```python
from build123d import *

# Parameters (mm, degrees)
F0_R     = 43.5
F0_R_2   = 41
F1_DEPTH = 14
F0_R_3   = 46.5412209473
F2_DEPTH = 2.5
F3_R     = 1.24999


# Not quite as in the source:
# - a fillet or chamfer is up to 0.001 mm smaller than in the source, because OpenCascade refuses the exact size


with BuildPart() as f1:
    # F0 (on Front) → F1 (new body)
    with BuildSketch(Plane.XZ):
        Circle(F0_R)
        Circle(F0_R_2, mode=Mode.SUBTRACT)
    extrude(amount=F1_DEPTH)

    # F0 (on Front) → F2 (join)
    with BuildSketch(Plane.XZ):
        Circle(F0_R_3)
        Circle(F0_R, mode=Mode.SUBTRACT)
    extrude(amount=F2_DEPTH)

    # F3 (radius 1.25 in the source; OpenCascade refuses exactly that, so slightly less here)
    f3_edges = [f1.edges().sort_by_distance(p)[0] for p in [
        (-46.541221, -2.5, 0),
        (-46.541221, 0, 0),
    ]]
    fillet(f3_edges, radius=F3_R)


solid = f1.part
```
Model file for the job. Use its own axes, mm. A direction names the side the tool comes from. Coordinates: 2 decimals unless noted, no trailing zeros. Loops run counter-clockwise (first coordinate to the right, second up) from the corner with the lowest first, then second, coordinate; pieces in that order, holes last. Notation, with made-up numbers: (-1, -15) - (56, -15) arc R13 cw to (56, -8) - close; hole circle Ø3 at (75, 36). An arc over 180 degrees is marked (long way). Write item = value, one per line. Start each with the question number.
Item 1: Saw through at C-C, the plane y = -9. List the corners of the cut face in (x, z).
Item 2: Pull direction Z, two halves, no side cores. Call faces 1 (the face through (-5.66, -8.17, 43.13)), 2 (the face through (-9, -7, -40)), 3 (the face through (-29.2, -14, 29.2)): +Z half, -Z half, draft (parallel to the pull), parting line (faces both ways), or undercut.
Item 3: Wall check: probe 1 along Z at (x, y) = (0, -9.75); probe 2 along Y at (x, z) = (-40.5, -16); probe 3 along X at (y, z) = (-9.5, 18). Give the ranges that are in metal, low to high. Write a range as [from, to].
Item 4: Drop flat-ended pins along their axis: pin 1 Ø4 at (x, y) = (4, -11) entering from +Z; pin 2 Ø10 at (x, z) = (22, 24.5) entering from +Y; pin 3 Ø6 at (y, z) = (-8, -9.5) entering from +X; pin 4 Ø4 at (y, z) = (-12, -5.5) entering from +X. Give the stop position or say it passes through.
Item 5: 3-axis set-ups, long thin cutter, end or side, ignore diameter. For faces 4 (the face through (-40.5, -2.5, 17)), 5 (the face through (-24, 0, 34)): which of +Z, -Z, +X, -X, +Y, -Y reach the whole face in a straight line?
Answers:
q1.outline = circle Ø87 at (0, 0); hole circle Ø82 at (0, 0)
q2.face_1 = parting line
q2.face_2 = undercut
q2.face_3 = draft
q3.probe_1 = [-43.5, -41], [41, 43.5]
q3.probe_2 = [-2.5, 0]
q3.probe_3 = [-39.6, -36.84], [36.84, 39.6]
q4.pin_1 = 43.45
q4.pin_2 = through
q4.pin_3 = 43.01
q4.pin_4 = 43.36
q5.face_4 = -Y
q5.face_5 = +Z, -Z, +X, -X, +Y
